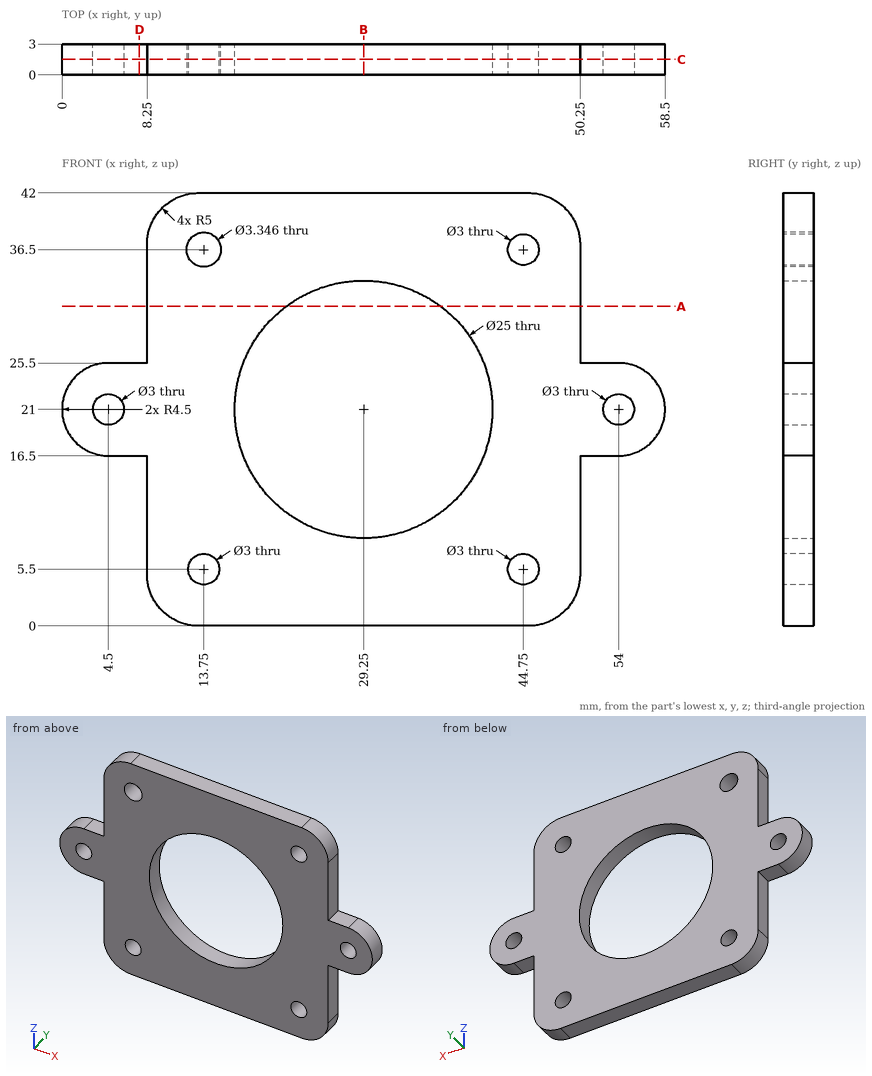
Geometry: see drawing. Coordinates: mm, zero at the bounding-box minimum. Coordinates: 2 decimals unless noted, no trailing zeros. Loops run counter-clockwise (first coordinate to the right, second up) from the corner with the lowest first, then second, coordinate; pieces in that order, holes last. Notation, with made-up numbers: M 50.5,36.5 L 104.5,36.5 A33 ccw 104.5,74.5 Z; hole C -16.5,25.25 d4. An arc over 180 degrees is marked long. Put each result on its own line as item: value. Start each with the question number.
1) Ray query, L1, parallel to X at y = 1.2, z = 21; L2, parallel to X at y = 1.4, z = 36.5; L3, parallel to Z at x = 13.75, y = 2.15. Return the intervals inside material, ascending. Write a range as from..to.
2) Cut plane C-C on y = 1.5. Return the cut outline in (x, z).
3) Cut plane A-A on z = 31. Return the cut outline in (x, y).
4) Cut plane D-D on x = 7.5. Return the cut outline in (y, z), then the cut area to 3 significant figures.
5) Contact query for flat-ended pins moving along their axis: pin 1 Ø0.9 at (y, z) = (2, 9) entering from -X; pin 2 Ø0.9 at (y, z) = (1.5, 29) entering from +X; pin 3 Ø1.5 at (x, y) = (52, 1) entering from -Z. Output: stop coordinate, or through.
6) Cut plane B-B on x = 29.25. Return the cut outline in (y, z), then the cut area to 3 significant figures.
The answers:
1. L1: x = 0..3, 6..16.75, 41.75..52.5, 55.5..58.5
1. L2: x = 8.25..12.08, 15.42..43.25, 46.25..50.25
1. L3: z = 0..4, 7..34.83, 38.17..42
2. outline: M 4.5,16.5 L 8.25,16.5 L 8.25,5 A5 ccw 13.25,0 L 45.25,0 A5 ccw 50.25,5 L 50.25,16.5 L 54,16.5 A4.5 ccw 54,25.5 L 50.25,25.5 L 50.25,37 A5 ccw 45.25,42 L 13.25,42 A5 ccw 8.25,37 L 8.25,25.5 L 4.5,25.5 A4.5 ccw Z; hole C 4.5,21 d3; hole C 13.75,36.5 d3.35; hole C 13.75,5.5 d3; hole C 29.25,21 d25; hole C 44.75,5.5 d3; hole C 44.75,36.5 d3; hole C 54,21 d3
3. outline: M 8.25,0 L 21.75,0 L 21.75,3 L 8.25,3 Z; M 36.75,0 L 50.25,0 L 50.25,3 L 36.75,3 Z
4. outline: M 0,16.5 L 3,16.5 L 3,25.5 L 0,25.5 Z
4. area: 27.0 mm²
5. pin 1: stops at x = 8.25
5. pin 2: stops at x = 50.25
5. pin 3: stops at z = 16.5
6. outline: M 0,0 L 3,0 L 3,8.5 L 0,8.5 Z; M 0,33.5 L 3,33.5 L 3,42 L 0,42 Z
6. area: 51.0 mm²
